Work out the finished part from the listing and answer in its coordinate system (mm). A direction names the side the tool comes from. Coordinates: 2 decimals unless noted, no trailing zeros. Loops run counter-clockwise (first coordinate to the right, second up) from the corner with the lowest first, then second, coordinate; pieces in that order, holes last. Notation, with made-up numbers: (16, 34.25) -> (49, 34.25) arc R19 cw to (49, 49.25) -> close; hole circle Ø9 at (39.25, -35). An arc over 180 degrees is marked (long way). Use a Markdown table: item, result.
from build123d import *

# Parameters (mm, degrees)
SKETCH1_R           = 40
SKETCH1_R_2         = 38
BOSS_EXTRUDE1_DEPTH = 250
SKETCH2_W           = 80
SKETCH2_H           = 20
CUT_EXTRUDE2_DEPTH  = 257.32011236


with BuildPart() as part:
    # Sketch1 → Boss-Extrude1 (new body)
    with BuildSketch(Plane(origin=(0, 0, 0), x_dir=(1, 0, 0), z_dir=(0, 1, 0))):
        with Locations(Location((0, 0, 0), (0, 0, 270))):
            Circle(SKETCH1_R)
        with Locations(Location((0, 0, 0), (0, 0, 270))):
            Circle(SKETCH1_R_2, mode=Mode.SUBTRACT)
    extrude(amount=BOSS_EXTRUDE1_DEPTH)

    # Sketch2 → Cut-Extrude2 (cut, through all)
    with BuildSketch(Plane.XY):
        with Locations((0, 160)):
            Rectangle(SKETCH2_W, SKETCH2_H)
    extrude(amount=CUT_EXTRUDE2_DEPTH, mode=Mode.SUBTRACT)


solid = part.part
Q1. Section A-A on z = -17.5 is taken. Determine the outline of the cut face in (x, y).
Solved:
| item | result |
|---|---|
| outline | (-35.97, 0) -> (-33.73, 0) -> (-33.73, 250) -> (-35.97, 250) -> close; (33.73, 0) -> (35.97, 0) -> (35.97, 250) -> (33.73, 250) -> close |
Q2. Section B-B on x = 0 is taken. Determine the outline of the cut face in (y, z).
Solved:
| item | result |
|---|---|
| outline | (0, -40) -> (250, -40) -> (250, -38) -> (0, -38) -> close; (0, 38) -> (150, 38) -> (150, 40) -> (0, 40) -> close; (170, 38) -> (250, 38) -> (250, 40) -> (170, 40) -> close |
Q3. For faces 4 (the flat face through (-14.6, 250, 35.4)), 5 (the flat face through (6, 150, 38)), determine the directions among +Z, -Z, +X, -X, +Y, -Y from which every point of the face is accessible in a straight line to the end or side of a thin tool.
Solved:
| item | result |
|---|---|
| face 4 | +Z, -Z, +X, -X, +Y |
| face 5 | +Z, +X, -X |
Q4. Determine the mould class of faces 1 (the flat face through (-14.6, 0, 35.4)), 2 (the cylindrical face through (1.671, 123.25, -37.963)), 3 (the cylindrical face through (1.76, 123.25, -39.96)) for opening direction X: pulls with the +X half, pulls with the -X half, needs draft (parallel to the pull), parting line crosses it, or undercut.
Solved:
| item | result |
|---|---|
| face 1 | needs draft |
| face 2 | undercut |
| face 3 | parting line crosses it |
Q5. Consider line 1 (X direction, y = 114, z = 0); line 2 (Y direction, x = -20, z = 34); line 3 (Z direction, x = -9, y = 129). Determine where each line is inside the solid, lowest interval first. Write a range as [from, to].
Solved:
| item | result |
|---|---|
| line 1 | [-40, -38], [38, 40] |
| line 2 | [0, 150], [170, 250] |
| line 3 | [-38.97, -36.92], [36.92, 38.97] |
Q6. Section C-C on z = 7 is taken. Determine the outline of the cut face in (x, y), and give its area (3 significant figures).
Solved:
| item | result |
|---|---|
| outline | (-39.38, 0) -> (-37.35, 0) -> (-37.35, 150) -> (-39.38, 150) -> close; (-39.38, 170) -> (-37.35, 170) -> (-37.35, 250) -> (-39.38, 250) -> close; (37.35, 0) -> (39.38, 0) -> (39.38, 150) -> (37.35, 150) -> close; (37.35, 170) -> (39.38, 170) -> (39.38, 250) -> (37.35, 250) -> close |
| area | 935 mm² |
Q7. Given pin 1 Ø12 at (x, z) = (-13, 28) entering from +Y; pin 2 Ø4 at (y, z) = (144.5, -22) entering from +X; pin 3 Ø6 at (x, y) = (30.5, 143) entering from +Z; pin 4 Ø5 at (x, y) = (-12, 89) entering from +Z, each flat-ended and moving along its own axis, determine where each tip first touches the part or whether it passes through.
Solved:
| item | result |
|---|---|
| pin 1 | through |
| pin 2 | x = 34.64 |
| pin 3 | z = 29.05 |
| pin 4 | z = 38.86 |
Q8. Section D-D on y = 152.5 is taken. Determine the outline of the cut face in (x, z), and give its area (3 significant figures).
Solved:
| item | result |
|---|---|
| outline | (-40, 0) arc R40 ccw to (40, 0) -> (38, 0) arc R38 cw to (-38, 0) -> close |
| area | 245 mm² |
